Here's the drawing with two shaded views (mm, measured from the low corner). I have some questions. Coordinates: 2 decimals unless noted, no trailing zeros. Loops run counter-clockwise (first coordinate to the right, second up) from the corner with the lowest first, then second, coordinate; pieces in that order, holes last. Notation, with made-up numbers: (-1, -7.75) -> (53, -7.75) arc R22 cw to (53, 15.25) -> close; hole circle Ø6 at (53.5, -24.5). An arc over 180 degrees is marked (long way). Answer as a JSON object with one key per item and string values. Group by question number.
Q1. I need wall thicknesses on line 1 (Y direction, x = 15, z = 19); line 2 (Y direction, x = 16.5, z = 18.5); line 3 (X direction, y = 11.5, z = 10). Which ranges of each line are inside material? Lowest first, please.
Q2. I want a section at A-A on z = 26.5. Write out the boundary of the cut face in (x, y) (1 decimal), then the cut area to 3 significant figures.
Q3. Thinking about a two-plate mould opening in Y: for the marked faces 1, 2 and 3, which applies, released by +Y, released by -Y, zero draft, split by the parting line, or undercut?
Q4. I'm going to push flat-ended pins straight in: pin 1 (1.4 mm diameter, centred on x = 0.5, z = 20.5, fed in from -Y); pin 2 (0.5 mm diameter, centred on y = 8.5, z = 28, fed in from +X) (3 decimals); pin 3 (6 mm diameter, centred on x = 13.5, y = 15, fed in from -Z); pin 4 (0.8 mm diameter, centred on y = 21.5, z = 20, fed in from -X) (3 decimals). Where does each tip first touch, or does it pass through?
Q5. I want a section at B-B on y = 15. Write out the boundary of the cut face in (x, z).
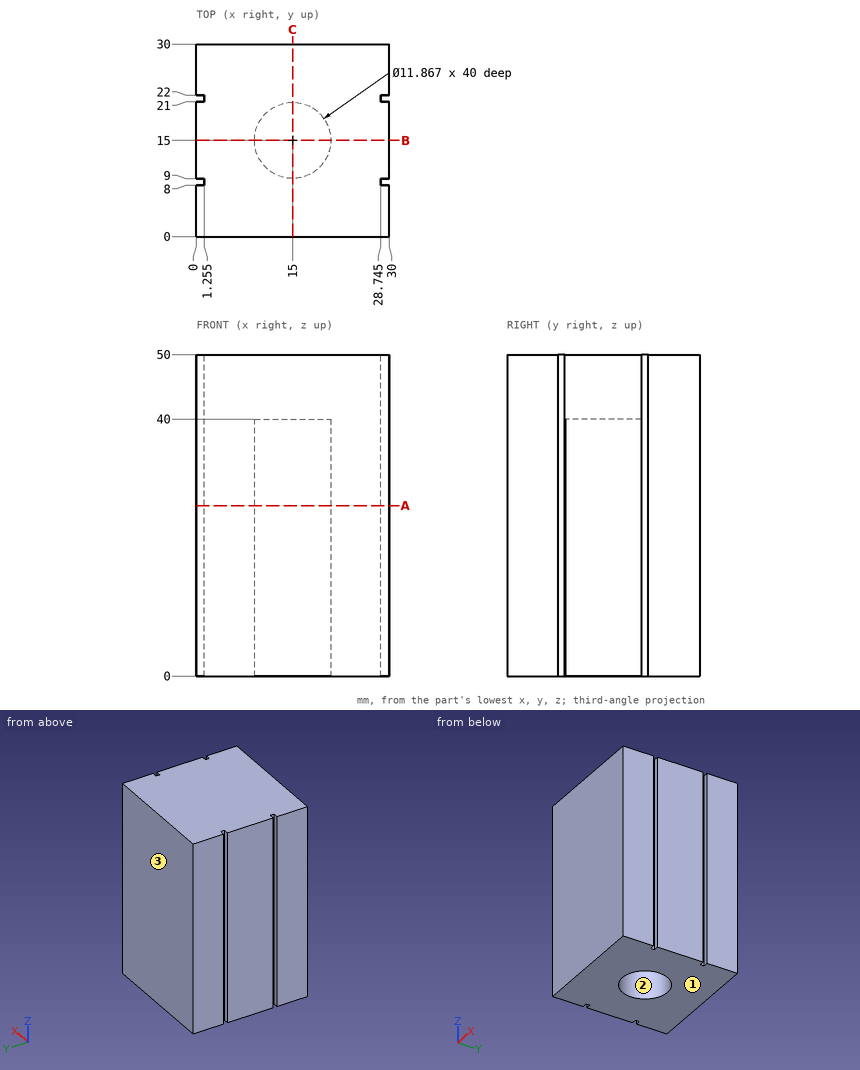
Result set:
{
 "1": {"line 1": "y = 0 to 9.07, 20.93 to 30", "line 2": "y = 0 to 9.26, 20.74 to 30", "line 3": "x = 0 to 10.21, 19.79 to 30"},
 "2": {"outline": "(0, 0) -> (30, 0) -> (30, 8) -> (28.7, 8) -> (28.7, 9) -> (30, 9) -> (30, 21) -> (28.7, 21) -> (28.7, 22) -> (30, 22) -> (30, 30) -> (0, 30) -> (0, 22) -> (1.3, 22) -> (1.3, 21) -> (0, 21) -> (0, 9) -> (1.3, 9) -> (1.3, 8) -> (0, 8) -> close; hole circle Ø11.9 at (15, 15)", "area": "784 mm²"},
 "3": {"face 1": "zero draft", "face 2": "undercut", "face 3": "released by +Y"},
 "4": {"pin 1": "stops at y = 0", "pin 2": "stops at x = 28.745", "pin 3": "stops at z = 40", "pin 4": "stops at x = 1.255"},
 "5": {"outline": "(0, 0) -> (9.07, 0) -> (9.07, 40) -> (20.93, 40) -> (20.93, 0) -> (30, 0) -> (30, 50) -> (0, 50) -> close"}
}
